Verification items for the finished model (mm, model axes). Face numbers are marked on the shaded views. A direction names the side the tool comes from. Give positions to 0.01 mm unless a question says otherwise; leave off trailing zeros. Order: outer loops, then holes, each group sorted by start corner. A loop starts at its lowest first (then second) coordinate and runs counter-clockwise, first axis right, second up.
from build123d import *

# Parameters (mm, degrees)
EXTRUS_O1_DEPTH = 19.6
EXTRUS_O2_DEPTH = 2.85
FILETE1_R       = 0.5
FILETE2_R       = 0.5
FILETE3_R       = 0.5
FILETE4_R       = 0.5
FILETE5_R       = 0.5
FILETE6_R       = 0.5
FILETE7_R       = 0.5
FILETE8_R       = 0.5
FILETE9_R       = 0.5
FILETE10_R      = 0.5
FILETE11_R      = 0.5
FILETE12_R      = 0.5
FILETE13_R      = 0.5
FILETE14_R      = 0.5
ESBO_O3_R       = 6.5
EXTRUS_O3_DEPTH = 2
ESBO_O4_R       = 4.45
EXTRUS_O4_DEPTH = 22
ESBO_O5_R       = 2.776577301
EXTRUS_O6_DEPTH = 10
FILETE15_R      = 0.5
FILETE16_R      = 0.5
FILETE17_R      = 0.5
FILETE18_R      = 0.5
FILETE19_R      = 0.5
FILETE20_R      = 0.5
FILETE21_R      = 0.5
FILETE22_R      = 0.5


with BuildPart() as part:
    # Esboço1 → Extrusão1 (new body)
    with BuildSketch(Plane(origin=(0, 0, 0), x_dir=(1, 0, 0), z_dir=(0, 1, 0))):
        Polygon((9.7, 12.3), (17.1, 12.3), (17.1, 9.8), (9.7, 9.8), (9.7, -16.5), (-29.1, -16.5), (-29.1, 9.8), (-36.5, 9.8), (-36.5, 12.3), (-29.1, 12.3), (-29.1, 16.5), (9.7, 16.5), align=None)
    extrude(amount=EXTRUS_O1_DEPTH)

    # Esboço2 → Extrusão2 (add)
    with BuildSketch(Plane(origin=(0, 0, -16.5), x_dir=(-1, 0, 0), z_dir=(0, 0, -1))):
        with BuildLine():
            Line((24.7, 19.4), (-0.981070844, 19.4))
            ThreePointArc((-0.981070844, 19.4), (-9.65, 9.8), (-0.981070844, 0.2))
            Line((-0.981070844, 0.2), (24.7, 0.2))
            Line((24.7, 0.2), (24.7, 6.356001076))
            ThreePointArc((24.7, 6.356001076), (26.318276276, 10.206001076), (24.7, 14.056001076))
            Line((24.7, 14.056001076), (24.7, 19.4))
        make_face()
    extrude(amount=EXTRUS_O2_DEPTH)

    # Filete1
    filete1_edges = [part.edges().sort_by_distance(p)[0] for p in [
        (17.1, 0, -11.05),
    ]]
    fillet(filete1_edges, radius=FILETE1_R)

    # Filete2
    filete2_edges = [part.edges().sort_by_distance(p)[0] for p in [
        (17.1, 19.6, -11.05),
    ]]
    fillet(filete2_edges, radius=FILETE2_R)

    # Filete3
    filete3_edges = [part.edges().sort_by_distance(p)[0] for p in [
        (-36.5, 0, -11.05),
    ]]
    fillet(filete3_edges, radius=FILETE3_R)

    # Filete4
    filete4_edges = [part.edges().sort_by_distance(p)[0] for p in [
        (-36.5, 19.6, -11.05),
    ]]
    fillet(filete4_edges, radius=FILETE4_R)

    # Filete5
    filete5_edges = [part.edges().sort_by_distance(p)[0] for p in [
        (-24.7, 0.2, -17.925),
    ]]
    fillet(filete5_edges, radius=FILETE5_R)

    # Filete6
    filete6_edges = [part.edges().sort_by_distance(p)[0] for p in [
        (-24.7, 19.4, -17.925),
    ]]
    fillet(filete6_edges, radius=FILETE6_R)

    # Filete7
    filete7_edges = [part.edges().sort_by_distance(p)[0] for p in [
        (-29.1, 0, 3.35),
    ]]
    fillet(filete7_edges, radius=FILETE7_R)

    # Filete8
    filete8_edges = [part.edges().sort_by_distance(p)[0] for p in [
        (-29.1, 19.6, 3.35),
    ]]
    fillet(filete8_edges, radius=FILETE8_R)

    # Filete9
    filete9_edges = [part.edges().sort_by_distance(p)[0] for p in [
        (9.7, 19.6, 3.35),
    ]]
    fillet(filete9_edges, radius=FILETE9_R)

    # Filete10
    filete10_edges = [part.edges().sort_by_distance(p)[0] for p in [
        (9.7, 0, 3.35),
    ]]
    fillet(filete10_edges, radius=FILETE10_R)

    # Filete11
    filete11_edges = [part.edges().sort_by_distance(p)[0] for p in [
        (-29.1, 0, -14.4),
    ]]
    fillet(filete11_edges, radius=FILETE11_R)

    # Filete12
    filete12_edges = [part.edges().sort_by_distance(p)[0] for p in [
        (-29.1, 19.6, -14.4),
    ]]
    fillet(filete12_edges, radius=FILETE12_R)

    # Filete13
    filete13_edges = [part.edges().sort_by_distance(p)[0] for p in [
        (9.7, 19.6, -14.4),
    ]]
    fillet(filete13_edges, radius=FILETE13_R)

    # Filete14
    filete14_edges = [part.edges().sort_by_distance(p)[0] for p in [
        (9.7, 0, -14.4),
    ]]
    fillet(filete14_edges, radius=FILETE14_R)

    # Esboço3 → Extrusão3 (add)
    with BuildSketch(Plane(origin=(0, 0, -19.35), x_dir=(-1, 0, 0), z_dir=(0, 0, -1))):
        with Locations((0.051438127, 9.966594638)):
            Circle(ESBO_O3_R)
    extrude(amount=EXTRUS_O3_DEPTH)

    # Esboço4 → Extrusão4 (cut)
    with BuildSketch(Plane(origin=(0, 0, -21.35), x_dir=(-1, 0, 0), z_dir=(0, 0, -1))):
        with Locations((0, 9.8)):
            Circle(ESBO_O4_R)
    extrude(amount=-EXTRUS_O4_DEPTH, mode=Mode.SUBTRACT)

    # Esboço5 → Extrusão6 (cut)
    with BuildSketch(Plane(origin=(0, 0, -12.3), x_dir=(-1, 0, 0), z_dir=(0, 0, -1))):
        with Locations((-14.650582931, 14.908902234)):
            Circle(ESBO_O5_R)
        with Locations((-14.650582931, 4.413440036)):
            Circle(ESBO_O5_R)
        with Locations((34.106114477, 14.908902234)):
            Circle(ESBO_O5_R)
        with Locations((34.106114477, 4.413440036)):
            Circle(ESBO_O5_R)
    extrude(amount=-EXTRUS_O6_DEPTH, mode=Mode.SUBTRACT)

    # Filete15
    filete15_edges = [part.edges().sort_by_distance(p)[0] for p in [
        (17.1, 5.721009358, -11.05),
    ]]
    fillet(filete15_edges, radius=FILETE15_R)

    # Filete16
    filete16_edges = [part.edges().sort_by_distance(p)[0] for p in [
        (17.1, 3.105870713, -11.05),
    ]]
    fillet(filete16_edges, radius=FILETE16_R)

    # Filete17
    filete17_edges = [part.edges().sort_by_distance(p)[0] for p in [
        (17.1, 16.216471557, -11.05),
    ]]
    fillet(filete17_edges, radius=FILETE17_R)

    # Filete18
    filete18_edges = [part.edges().sort_by_distance(p)[0] for p in [
        (17.1, 13.601332911, -11.05),
    ]]
    fillet(filete18_edges, radius=FILETE18_R)

    # Filete19
    filete19_edges = [part.edges().sort_by_distance(p)[0] for p in [
        (-36.5, 16.315562682, -11.05),
    ]]
    fillet(filete19_edges, radius=FILETE19_R)

    # Filete20
    filete20_edges = [part.edges().sort_by_distance(p)[0] for p in [
        (-36.5, 13.502241787, -11.05),
    ]]
    fillet(filete20_edges, radius=FILETE20_R)

    # Filete21
    filete21_edges = [part.edges().sort_by_distance(p)[0] for p in [
        (-36.5, 3.006779588, -11.05),
    ]]
    fillet(filete21_edges, radius=FILETE21_R)

    # Filete22
    filete22_edges = [part.edges().sort_by_distance(p)[0] for p in [
        (-36.5, 5.820100483, -11.05),
    ]]
    fillet(filete22_edges, radius=FILETE22_R)


solid = part.part
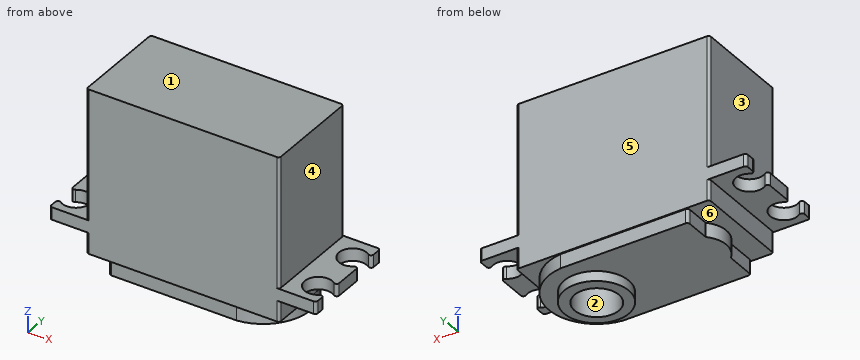
(1) Go/stop test with flat-tipped pins: pin 1 (0.9 mm diameter, centred on x = -9, z = -17.5, fed in from +Y); pin 2 (1.4 mm diameter, centred on x = -6.5, z = -18.5, fed in from -Y); pin 3 (2.5 mm diameter, centred on x = -34, y = 6.5, fed in from -Z); pin 4 (5 mm diameter, centred on x = 14.65, y = 4.41, fed in from +Z). Record where each tip stops, or that it passes through.
Solved:
pin 1: stops at y = 19.4
pin 2: stops at y = 0.2
pin 3: stops at z = -12.3
pin 4: passes through
(2) Set-up check for the marked faces 4, 5 and 6: record each of +Z, -Z, +X, -X, +Y, -Y from which the full face is reachable in a straight line by a thin tool's end or side.
Solved:
face 4: +Z, +X, +Y, -Y
face 5: +Z, -Z, +X, -X, +Y
face 6: -Z
(3) Scan lines: line 1 (Y direction, x = 0, z = -4.25); line 2 (Z direction, x = -25.5, y = 3.75); line 3 (X direction, y = 4.25, z = -9). Record each from-to range of solid material in increasing order.
Solved:
line 1: y = 0 to 5.35, 14.25 to 19.6
line 2: z = -16.5 to 16.5
line 3: x = -29.1 to 9.7
(4) Section check D-D, the plane x = 0. Enter the section's corners in (y, z).
Solved:
outline: (0, -16.5) - (0.2, -16.5) - (0.2, -19.35) - (3.47, -19.35) - (3.47, -21.35) - (5.35, -21.35) - (5.35, 0.65) - (14.25, 0.65) - (14.25, -21.35) - (16.47, -21.35) - (16.47, -19.35) - (19.4, -19.35) - (19.4, -16.5) - (19.6, -16.5) - (19.6, 16.5) - (0, 16.5) - close
(5) Section check A-A, the plane z = 3. Enter the section's corners in (x, y), then the cut area to 3 significant figures.
Solved:
outline: (-29.1, 0.5) arc R0.5 ccw to (-28.6, 0) - (9.2, 0) arc R0.5 ccw to (9.7, 0.5) - (9.7, 19.1) arc R0.5 ccw to (9.2, 19.6) - (-28.6, 19.6) arc R0.5 ccw to (-29.1, 19.1) - close
area: 760 mm2
(6) Section check C-C, the plane x = 8. Enter the section's corners in (y, z), then the cut area to 3 significant figures.
Solved:
outline: (0, -16.5) - (4.4, -16.5) - (4.4, -19.35) - (15.2, -19.35) - (15.2, -16.5) - (19.6, -16.5) - (19.6, 16.5) - (0, 16.5) - close
area: 678 mm2
(7) Section check B-B, the plane y = 8.5. Enter the section's corners in (x, z), then the cut area to 3 significant figures.
Solved:
outline: (-36.5, -12.3) - (-29.1, -12.3) - (-29.1, -16.5) - (-26.04, -16.5) - (-26.04, -19.35) - (-6.38, -19.35) - (-6.38, -21.35) - (-4.26, -21.35) - (-4.26, 0.65) - (4.26, 0.65) - (4.26, -21.35) - (6.28, -21.35) - (6.28, -19.35) - (9.56, -19.35) - (9.56, -16.5) - (9.7, -16.5) - (9.7, -12.3) - (17.1, -12.3) - (17.1, -9.8) - (9.7, -9.8) - (9.7, 16.5) - (-29.1, 16.5) - (-29.1, -9.8) - (-36.5, -9.8) - close
area: 1,260 mm2
(8) Release check for a two-part mould opening along X. For the marked faces 1, 2 and 3 record: pulls with the +X half, pulls with the -X half, needs draft (parallel to the pull), parting line crosses it, or undercut.
Solved:
face 1: needs draft
face 2: undercut
face 3: pulls with the -X half
